Read the model definition and answer for the solid it produces. Units are mm, in the model's axes. Coordinates: 2 decimals unless noted, no trailing zeros. Order: outer loops, then holes, each group sorted by start corner. A loop starts at its lowest first (then second) coordinate and runs counter-clockwise, first axis right, second up.
```python
from build123d import *

# Parameters (mm, degrees)
SKETCH_1_R           = 210
EXTRUDE_1_DEPTH      = 10
SKETCH_2_R           = 75
CUT_EXTRUDE_1_DEPTH  = 10
SKETCH_4_R           = 82.197423103
CUT_EXTRUDE_3_DEPTH  = 10
SKETCH_5_R           = 232.576786868
SKETCH_5_R_2         = 183.037626036
CUT_EXTRUDE_4_DEPTH  = 10
CUT_EXTRUDE_6_DEPTH  = 10
CUT_EXTRUDE_7_DEPTH  = 10
EXTRUDE_2_DEPTH      = 10
SKETCH_8_R           = 3.37024185
CUT_EXTRUDE_9_DEPTH  = 10
EXTRUDE_START        = -10
EXTRUDE_3_DEPTH      = 10
SKETCH_10_R          = 221.118951793
SKETCH_10_R_2        = 189.34656242
CUT_EXTRUDE_10_DEPTH = 20
SKETCH_11_R          = 238.000555744
SKETCH_11_R_2        = 183.483177488
CUT_EXTRUDE_11_DEPTH = 20


with BuildPart() as part:
    # 草图1 → 凸台-拉伸1 (new body)
    with BuildSketch(Plane(origin=(0, 0, 0), x_dir=(1, 0, 0), z_dir=(0, 1, 0))):
        with Locations(Location((0, 0, 0), (0, 0, 270))):
            Circle(SKETCH_1_R)
    extrude(amount=EXTRUDE_1_DEPTH)

    # 草图2 → 切除-拉伸1 (cut)
    with BuildSketch(Plane(origin=(0, 10, 0), x_dir=(1, 0, 0), z_dir=(0, 1, 0))):
        with Locations(Location((0, 0, 0), (0, 0, 270))):
            Circle(SKETCH_2_R)
    extrude(amount=-CUT_EXTRUDE_1_DEPTH, mode=Mode.SUBTRACT)

    # 草图4 → 切除-拉伸3 (cut)
    with BuildSketch(Plane(origin=(0, 10, 0), x_dir=(1, 0, 0), z_dir=(0, 1, 0))):
        with Locations(Location((0, 0, 0), (0, 0, 270))):
            Circle(SKETCH_4_R)
    extrude(amount=-CUT_EXTRUDE_3_DEPTH, mode=Mode.SUBTRACT)

    # 草图5 → 切除-拉伸4 (cut)
    with BuildSketch(Plane(origin=(0, 10, 0), x_dir=(1, 0, 0), z_dir=(0, 1, 0))):
        Circle(SKETCH_5_R)
        with Locations(Location((0, 0, 0), (0, 0, 270))):
            Circle(SKETCH_5_R_2, mode=Mode.SUBTRACT)
    extrude(amount=-CUT_EXTRUDE_4_DEPTH, mode=Mode.SUBTRACT)

    # 草图3 → 切除-拉伸6 (cut)
    with BuildSketch(Plane(origin=(0, 10, 0), x_dir=(1, 0, 0), z_dir=(0, 1, 0))):
        Polygon((-218.107078413, -133.413550562), (-168.78547064, -202.149571439), (-50, -50), (50, -50), (168.78547064, -202.149571439), (64.609548257, -313.747882065), (267.248585971, -202.149571439), (429.751389162, 108.172046702), (-16.641853339, 302.979624022), (-278.723850855, 176.468454352), align=None)
    extrude(amount=-CUT_EXTRUDE_6_DEPTH, mode=Mode.SUBTRACT)

    # 草图6 → 切除-拉伸7 (cut)
    with BuildSketch(Plane(origin=(0, 10, 0), x_dir=(1, 0, 0), z_dir=(0, 1, 0))):
        Polygon((0, 0), (0, -233.405297089), (-177.211837764, -160.795172893), (-110.712466595, -38.220656306), align=None)
    extrude(amount=-CUT_EXTRUDE_7_DEPTH, mode=Mode.SUBTRACT)

    # 草图7 → 凸台-拉伸2 (add)
    with BuildSketch(Plane(origin=(0, 10, 0), x_dir=(1, 0, 0), z_dir=(0, 1, 0))):
        with BuildLine():
            Line((0, -131.161321566), (0, -190))
            ThreePointArc((0, -190), (65.897168622, -178.206518308), (123.6137367, -144.290138606))
            Line((123.6137367, -144.290138606), (94.010463478, -106.371988266))
            Line((94.010463478, -106.371988266), (0, -131.161321566))
        make_face()
    extrude(amount=-EXTRUDE_2_DEPTH)

    # 草图8 → 切除-拉伸9 (cut)
    with BuildSketch(Plane(origin=(0, 10, 0), x_dir=(1, 0, 0), z_dir=(0, 1, 0))):
        with Locations(Location((72.297266291, -98.948546348, 0), (0, 0, 270))):
            Circle(SKETCH_8_R)
    extrude(amount=-CUT_EXTRUDE_9_DEPTH, mode=Mode.SUBTRACT)

    # 草图9 → 凸台-拉伸3 (add)
    with BuildSketch(Plane.XZ.offset(EXTRUDE_START)):
        with BuildLine():
            Line((-72.52965516, 175.611642901), (-31.37763554, 75.972760596))
            ThreePointArc((-31.37763554, 75.972760596), (-15.994549348, 80.626241112), (0, 82.197423103))
            Line((0, 82.197423103), (0, 190))
            ThreePointArc((0, 190), (-36.971528565, 186.36820028), (-72.52965516, 175.611642901))
        make_face()
    extrude(amount=EXTRUDE_3_DEPTH)

    # 草图10 → 切除-拉伸10 (cut)
    with BuildSketch(Plane.XZ):
        with Locations((6.928171241, 3.379528268)):
            Circle(SKETCH_10_R)
        Circle(SKETCH_10_R_2, mode=Mode.SUBTRACT)
    extrude(amount=-CUT_EXTRUDE_10_DEPTH, mode=Mode.SUBTRACT)

    # 草图11 → 切除-拉伸11 (cut)
    with BuildSketch(Plane.XZ):
        with Locations((0, 17.732727097)):
            Circle(SKETCH_11_R)
        Circle(SKETCH_11_R_2, mode=Mode.SUBTRACT)
    extrude(amount=-CUT_EXTRUDE_11_DEPTH, mode=Mode.SUBTRACT)


solid = part.part
```
1) A cutting plane is placed at A-A, the plane z = 99.5. Determine the outline of the cut face in (x, y), and give its area (3 significant figures).
A:
outline: (-41.09, 0) - (68.97, 0) - (68.97, 10) - (-41.09, 10) - close; (75.62, 0) - (88.65, 0) - (88.65, 10) - (75.62, 10) - close
area: 1,230 mm2
2) A cutting plane is placed at C-C, the plane x = -34.5. Determine the outline of the cut face in (y, z).
A:
outline: (0, 83.53) - (10, 83.53) - (10, 180.21) - (0, 180.21) - close
3) Straight lines are drawn through the part: line 1 (Z direction, x = -26.5, y = 3.5); line 2 (Z direction, x = 86, y = 3.25); line 3 (X direction, y = 1, z = 124.5). For each, find the intervals that lie inside material, in ascending order.
A:
line 1: z = 77.81 to 181.56
line 2: z = 96.11 to 162.08
line 3: x = -51.42 to 108.16
4) Flat-ended cylindrical pins translate along their axes: pin 1 Ø3 at (y, z) = (9, 131.5) entering from +X; pin 2 Ø6 at (x, y) = (82.5, 7) entering from -Z; pin 3 Ø1.5 at (y, z) = (1, 71.5) entering from +X. Find the tip coordinate at first contact, or state that the pin passes through.
A:
pin 1: stops at x = 114.8
pin 2: stops at z = 87.79
pin 3: stops at x = 67.37
5) Determine the mould class of faces 1 (the flat face through (-50.98, 5.07, 123.44)), 2 (the cylindrical face through (30.476, 4.93, 180.934)), 3 (the cylindrical face through (70.25, 5.07, 96.27)) for opening direction X: pulls with the +X half, pulls with the -X half, needs draft (parallel to the pull), parting line crosses it, or undercut.
A:
face 1: pulls with the -X half
face 2: parting line crosses it
face 3: undercut
6) A cutting plane is placed at D-D, the plane z = 125. Determine the outline of the cut face in (x, y), and give its area (3 significant figures).
A:
outline: (-51.63, 0) - (108.55, 0) - (108.55, 10) - (-51.63, 10) - close
area: 1,600 mm2
7) A cutting plane is placed at B-B, the plane y = 3. Determine the outline of the cut face in (x, z), and give its area (3 significant figures).
A:
outline: (-70.04, 169.59) - (-31.38, 75.97) arc R82.2 cw to (57.11, 59.11) - (119.6, 139.15) arc R183.48 ccw to start; hole circle Ø6.74 at (72.3, 98.95)
area: 15,000 mm2
